from build123d import *

# Parameters (mm, degrees)
SKETCH1_W           = 25.4
SKETCH1_H           = 6.35
SKETCH1_W_2         = 6.35
SKETCH1_H_2         = 31.75
BOSS_EXTRUDE1_DEPTH = 50.8
CUT_EXTRUDE1_REACH  = 8.35
SKETCH2_R           = 6.3627
CUT_EXTRUDE2_REACH  = 8.35
SKETCH3_R           = 3.96875


with BuildPart() as part:
    # Sketch1 → Boss-Extrude1 (new body)
    with BuildSketch(Plane(origin=(0, 0, 0), x_dir=(0, 0, -1), z_dir=(1, 0, 0))):
        with Locations((-19.05, 3.175)):
            Rectangle(SKETCH1_W, SKETCH1_H)
        with Locations((-3.175, 15.875)):
            Rectangle(SKETCH1_W_2, SKETCH1_H_2)
    extrude(amount=BOSS_EXTRUDE1_DEPTH)

    # Sketch2 → Cut-Extrude1 (cut, up to next)
    with BuildSketch(Plane.XY.offset(6.35), mode=Mode.PRIVATE) as cut_extrude1_sk1:
        with Locations((25.4, 20.32)):
            Circle(SKETCH2_R)
    cut_extrude1_tool1 = extrude(cut_extrude1_sk1.sketch, amount=-CUT_EXTRUDE1_REACH, mode=Mode.PRIVATE) & part.part
    add(cut_extrude1_tool1.solids().sort_by_distance((25.4, 20.32, 6.35))[0], mode=Mode.SUBTRACT)

    # Sketch3 → Cut-Extrude2 (cut, up to next)
    with BuildSketch(Plane(origin=(0, 6.35, 0), x_dir=(1, 0, 0), z_dir=(0, 1, 0)), mode=Mode.PRIVATE) as cut_extrude2_sk1:
        with Locations((12.7, -19.05)):
            Circle(SKETCH3_R)
    cut_extrude2_tool1 = extrude(cut_extrude2_sk1.sketch, amount=-CUT_EXTRUDE2_REACH, mode=Mode.PRIVATE) & part.part
    add(cut_extrude2_tool1.solids().sort_by_distance((12.7, 6.35, 19.05))[0], mode=Mode.SUBTRACT)
    # Sketch3 → Cut-Extrude2 (cut, up to next)
    with BuildSketch(Plane(origin=(0, 6.35, 0), x_dir=(1, 0, 0), z_dir=(0, 1, 0)), mode=Mode.PRIVATE) as cut_extrude2_sk2:
        with Locations((38.1, -19.05)):
            Circle(SKETCH3_R)
    cut_extrude2_tool2 = extrude(cut_extrude2_sk2.sketch, amount=-CUT_EXTRUDE2_REACH, mode=Mode.PRIVATE) & part.part
    add(cut_extrude2_tool2.solids().sort_by_distance((38.1, 6.35, 19.05))[0], mode=Mode.SUBTRACT)


solid = part.part
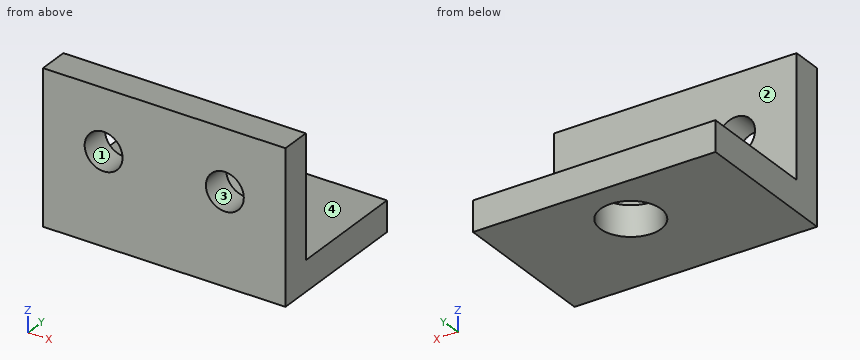
Verification items for the finished model (mm, model axes). Face numbers are marked on the shaded views. Give positions to 0.01 mm unless a question says otherwise; leave off trailing zeros. Write each loop counter-clockwise with the first axis right and the second up, starting at its lowest first coordinate (ties: lowest second). Pieces come first, ordered by that corner, then holes.
(1) Cross-section at A-A (x = 38.1). Enter the section's corners in (y, z).
(2) Gauge pin test, flat ends, axial feed: pin 1 (12.5 mm diameter, centred on x = 30.5, y = 22.5, fed in from +Z); pin 2 (8 mm diameter, centred on x = 12, y = 18.5, fed in from +Z); pin 3 (4 mm diameter, centred on x = 24.5, z = 24, fed in from +Y); pin 4 (5 mm diameter, centred on x = 38.1, z = 19.05, fed in from +Y). Record the tip position at first contact, or that the pin passes through.
(3) Cross-section at B-B (y = 20.32). Enter the section's corners in (x, z), plus the area to 3 significant figures.
(4) Mould release check, pull along Z, two halves, no side actions. Record for the marked faces 1, 2, 3 and 4: +Z half, -Z half, draft (parallel to the pull), parting line (faces both ways), or undercut.
(5) Material ranges on line 1 (X direction, y = 1, z = 19); line 2 (Z direction, x = 38.1, y = 2.5); line 3 (Y direction, x = 25.4, z = 2), recorded low to high.
(6) Cross-section at D-D (x = 25.4). Enter the section's corners in (y, z), plus the area to 3 significant figures.
(7) Cross-section at C-C (z = 19.05). Enter the section's corners in (x, y).
Worked out:
1. outline: (0, 0) - (31.75, 0) - (31.75, 6.35) - (6.35, 6.35) - (6.35, 15.08) - (0, 15.08) - close; (0, 23.02) - (6.35, 23.02) - (6.35, 31.75) - (0, 31.75) - close
2. pin 1: stops at z = 6.35
2. pin 2: stops at z = 6.35
2. pin 3: stops at y = 6.35
2. pin 4: passes through
3. outline: (0, 0) - (19.04, 0) - (19.04, 6.35) - (0, 6.35) - close; (31.76, 0) - (50.8, 0) - (50.8, 6.35) - (31.76, 6.35) - close
3. area: 242 mm2
4. face 1: undercut
4. face 2: draft
4. face 3: undercut
4. face 4: +Z half
5. line 1: x = 0 to 8.73, 16.67 to 34.13, 42.07 to 50.8
5. line 2: z = 0 to 15.08, 23.02 to 31.75
5. line 3: y = 0 to 13.96, 26.68 to 31.75
6. outline: (0, 0) - (13.96, 0) - (13.96, 6.35) - (6.35, 6.35) - (6.35, 31.75) - (0, 31.75) - close; (26.68, 0) - (31.75, 0) - (31.75, 6.35) - (26.68, 6.35) - close
6. area: 282 mm2
7. outline: (0, 0) - (8.73, 0) - (8.73, 6.35) - (0, 6.35) - close; (16.67, 0) - (34.13, 0) - (34.13, 6.35) - (16.67, 6.35) - close; (42.07, 0) - (50.8, 0) - (50.8, 6.35) - (42.07, 6.35) - close
